Build history of the part. All positions in model axes, mm. A direction names the side the tool comes from. Give positions to 0.01 mm unless a question says otherwise; leave off trailing zeros. Loops run counter-clockwise (first coordinate to the right, second up) from the corner with the lowest first, then second, coordinate; pieces in that order, holes last.
1) 3-axis set-ups, long thin cutter, end or side, ignore diameter. For faces 1 (the flat face through (36, 11.906, -16)), 2 (the cylindrical face through (36.396, 11.33, -13.933)): which of +Z, -Z, +X, -X, +Y, -Y reach the whole face in a straight line?
2) Flat gauge pins, fed straight in: P1, Ø2, axis at x = 49, z = 4, coming from the -Y side; P2, Ø8, axis at x = 65.5, z = -2, coming from the +Y side. Where does each tip first touch, or does it go through?
3) Band-saw the part on A-A on z = 5.5. List the corners of the cut face in (x, y) (1 decimal).
4) Two-plate mould, pull along Z, no slides. Class faces 3 (the flat face through (0, 3, 0)), 4 (the cylindrical face through (36.396, 11.299, 13.902)), 5 (the flat face through (37, 6, -17.519)): +Z half, -Z half, draft (parallel to the pull), parting line (faces both ways), or undercut.
5) Wall check: line 1 (Z direction, x = 26, y = 10); line 2 (Y direction, x = 14.5, z = 8); line 3 (Z direction, x = 16, y = 5). Give the ranges that are in metal, low to high.
```python
from build123d import *

# Parameters (mm, degrees)
BOSS_EXTRUDE1_DEPTH = 73.824999924
SKETCH2_W           = 5.5
SKETCH2_H           = 11.90625
CUT_EXTRUDE1_DEPTH  = 77


with BuildPart() as part:
    # Sketch1 → Boss-Extrude1 (new body)
    with BuildSketch(Plane(origin=(0, 0, 0), x_dir=(0, 0, -1), z_dir=(1, 0, 0))):
        with BuildLine():
            Line((-16.615833333, 11.90625), (-23.01875, 11.90625))
            Line((-23.01875, 11.90625), (-23.01875, 0))
            Line((-23.01875, 0), (23.01875, 0))
            Line((23.01875, 0), (23.01875, 11.90625))
            Line((23.01875, 11.90625), (16.615833333, 11.90625))
            Line((16.615833333, 11.90625), (15.345833333, 11.90625))
            ThreePointArc((15.345833333, 11.90625), (13.917616741, 11.314663318), (13.326030059, 9.886446726))
            add(Edge.make_bspline(
                [(13.328163425, 9.793638273), (13.326964681, 9.82406182), (13.32624931, 9.854992294), (13.326030059, 9.886446726)],
                knots=[0.989153926, 0.989153926, 0.989153926, 0.989153926, 1, 1, 1, 1], degree=3))
            add(Edge.make_bspline(
                [(13.44097879, 4.843193137), (13.756839485, 4.900565232), (14.289482388, 5.115085376), (14.924667677, 5.682716987), (15.305824568, 6.321722829), (15.357243262, 7.163342963), (14.243691121, 8.123322783), (13.37079951, 8.71155514), (13.328163425, 9.793638273)],
                knots=[0.001929893, 0.001929893, 0.001929893, 0.001929893, 0.146224432, 0.253988964, 0.379668219, 0.474367728, 0.603388454, 0.989153926, 0.989153926, 0.989153926, 0.989153926], degree=3))
            ThreePointArc((13.44097879, 4.843193137), (13.125958752, 4.782754037), (12.805833333, 4.7625))
            Line((12.805833333, 4.7625), (-12.805833333, 4.7625))
            ThreePointArc((-12.805833333, 4.7625), (-13.125958752, 4.782754037), (-13.44097879, 4.843193137))
            add(Edge.make_bspline(
                [(-13.44097879, 4.843193137), (-13.756839485, 4.900565232), (-14.289482388, 5.115085376), (-14.924667677, 5.682716987), (-15.305824568, 6.321722829), (-15.357243262, 7.163342963), (-14.243691121, 8.123322783), (-13.37079951, 8.71155514), (-13.328163425, 9.793638273)],
                knots=[0.001929893, 0.001929893, 0.001929893, 0.001929893, 0.146224432, 0.253988964, 0.379668219, 0.474367728, 0.603388454, 0.989153926, 0.989153926, 0.989153926, 0.989153926], degree=3))
            add(Edge.make_bspline(
                [(-13.328163425, 9.793638273), (-13.326964681, 9.82406182), (-13.32624931, 9.854992294), (-13.326030059, 9.886446726)],
                knots=[0.989153926, 0.989153926, 0.989153926, 0.989153926, 1, 1, 1, 1], degree=3))
            ThreePointArc((-13.326030059, 9.886446726), (-13.917616741, 11.314663318), (-15.345833333, 11.90625))
            Line((-15.345833333, 11.90625), (-16.615833333, 11.90625))
        make_face()
    extrude(amount=BOSS_EXTRUDE1_DEPTH)

    # Sketch2 → Cut-Extrude1 (cut)
    with BuildSketch(Plane(origin=(73.824999924, 0, 0), x_dir=(0, 0, -1), z_dir=(1, 0, 0))):
        with Locations((-20.26875, 5.953125)):
            Rectangle(SKETCH2_W, SKETCH2_H)
        with Locations((20.26875, 5.953125)):
            Rectangle(SKETCH2_W, SKETCH2_H)
    extrude(amount=-CUT_EXTRUDE1_DEPTH, mode=Mode.SUBTRACT)


solid = part.part
```
Findings below:
1. face 1: +Z, -Z, +X, -X, +Y
1. face 2: +X, -X, +Y
2. P1: stops at y = 0
2. P2: stops at y = 4.76
3. outline: (0, 0) - (73.8, 0) - (73.8, 4.8) - (0, 4.8) - close
4. face 3: draft
4. face 4: undercut
4. face 5: -Z half
5. line 1: z = -17.52 to -13.33, 13.33 to 17.52
5. line 2: y = 0 to 4.76
5. line 3: z = -17.52 to -13.96, 13.96 to 17.52
